Source: three-view drawing plus pictorial views. Frame: mm from the lowest corner of the part. Give positions to 0.01 mm unless a question says otherwise; leave off trailing zeros. Order: outer loops, then holes, each group sorted by start corner. A loop starts at its lowest first (then second) coordinate and runs counter-clockwise, first axis right, second up. Notation, with made-up numbers: (63.5, -15) -> (122.5, -15) arc R30 ccw to (122.5, 13) -> close; hole circle Ø1 at (-10, 60). An arc over 180 degrees is marked (long way). Answer in a Markdown table with one row per item.
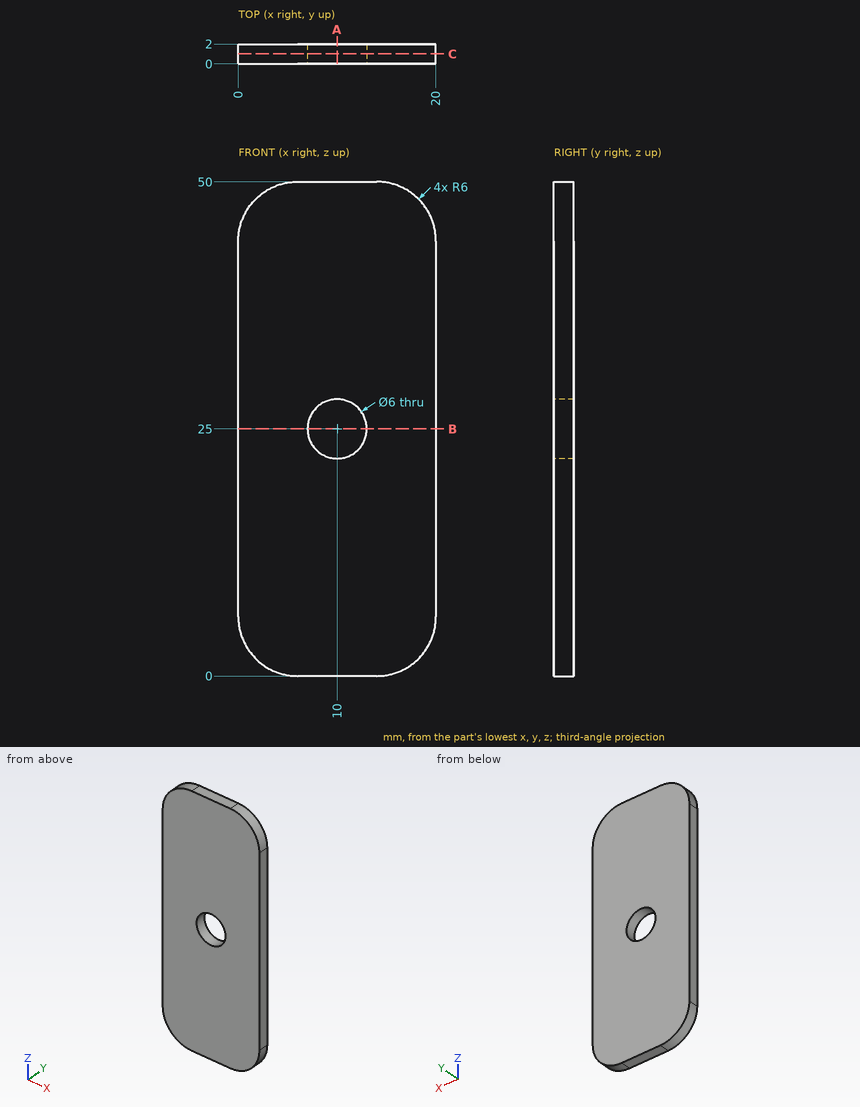
(1) Section query C-C (y = 1). Return the cut outline in (x, z), plus the area to 3 significant figures.
A:
| item | result |
|---|---|
| outline | (0, 6) arc R6 ccw to (6, 0) -> (14, 0) arc R6 ccw to (20, 6) -> (20, 44) arc R6 ccw to (14, 50) -> (6, 50) arc R6 ccw to (0, 44) -> close; hole circle Ø6 at (10, 25) |
| area | 941 mm^2 |
(2) Section query B-B (z = 25). Return the cut outline in (x, y).
A:
| item | result |
|---|---|
| outline | (0, 0) -> (7, 0) -> (7, 2) -> (0, 2) -> close; (13, 0) -> (20, 0) -> (20, 2) -> (13, 2) -> close |
(3) Ray query, probe 1 along Z at (x, y) = (10, 0.85); probe 2 along X at (y, z) = (1.35, 25); probe 3 along X at (y, z) = (0.6, 26). Return the intervals inside material, ascending.
A:
| item | result |
|---|---|
| probe 1 | z = 0 to 22, 28 to 50 |
| probe 2 | x = 0 to 7, 13 to 20 |
| probe 3 | x = 0 to 7.17, 12.83 to 20 |
(4) Section query A-A (x = 10). Return the cut outline in (y, z), plus the area to 3 significant figures.
A:
| item | result |
|---|---|
| outline | (0, 0) -> (2, 0) -> (2, 22) -> (0, 22) -> close; (0, 28) -> (2, 28) -> (2, 50) -> (0, 50) -> close |
| area | 88.0 mm^2 |
